Design review of the part built by this model. Coordinates are the model's own, in mm. Face numbers are marked on the shaded views. A direction names the side the tool comes from. Round coordinates to 2 decimals unless told otherwise and drop trailing zeros. Loops run counter-clockwise (first coordinate to the right, second up) from the corner with the lowest first, then second, coordinate; pieces in that order, holes last. Notation, with made-up numbers: (70.25, 68) -> (81.25, 68) arc R25 ccw to (81.25, 94) -> close; hole circle Ø1 at (20.5, 49.25). An arc over 180 degrees is marked (long way). Use a Markdown table: item, result. Add a question column.
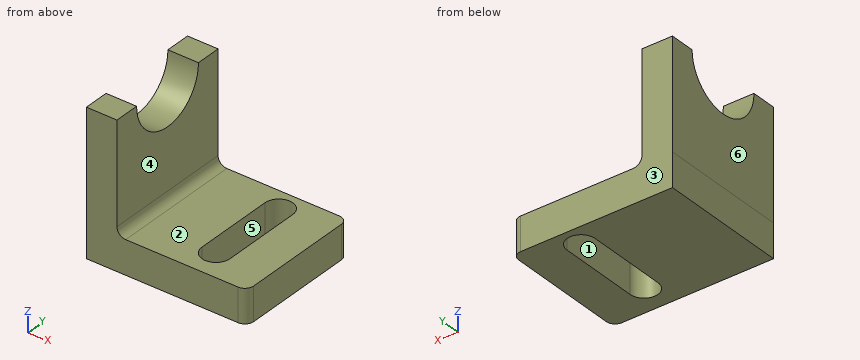
from build123d import *

# Parameters (mm, degrees)
F0_W     = 17.553337
F0_H     = 62.748581
F1_DEPTH = 75
F2_R     = 22.940745
F3_DEPTH = 25
F5_DEPTH = 19.308256
F6_R     = 5
F7_R     = 5


with BuildPart() as f1:
    # F0 (on Front) → F1 (new body)
    with BuildSketch(Plane.XZ):
        Polygon((-46.077821, -9.653628), (46.077821, -9.653628), (46.077821, 9.653628), (-28.524484, 9.653628), (-46.077821, 9.653628), align=None)
        with Locations((-37.301153, 41.027918)):
            Rectangle(F0_W, F0_H)
    extrude(amount=F1_DEPTH)

    # F2 (on face) → F3 (cut)
    with BuildSketch(Plane.YZ.offset(-28.524484)):
        with Locations((-37.5, 72.402209)):
            Circle(F2_R)
    extrude(amount=-F3_DEPTH, mode=Mode.SUBTRACT)

    # F4 (on face) → F5 (cut, through all)
    with BuildSketch(Plane.XY.offset(9.653628)):
        with BuildLine():
            Line((7.655139, -12.002843), (7.655139, -58.650463))
            ThreePointArc((7.655139, -58.650463), (15.655139, -66.650463), (23.655139, -58.650463))
            Line((23.655139, -58.650463), (23.655139, -12.002843))
            ThreePointArc((23.655139, -12.002843), (15.655139, -4.002843), (7.655139, -12.002843))
        make_face()
    extrude(amount=-F5_DEPTH, mode=Mode.SUBTRACT)

    # F6
    f6_edges = [f1.edges().sort_by_distance(p)[0] for p in [
        (46.077821, -75, 0),
        (46.077821, 0, 0),
    ]]
    fillet(f6_edges, radius=F6_R)

    # F7
    f7_edges = [f1.edges().sort_by_distance(p)[0] for p in [
        (-28.524484, -37.5, 9.653628),
    ]]
    fillet(f7_edges, radius=F7_R)


solid = f1.part
1. For the marked faces 1, 2 and 3, list the 3-axis set-ups (+Z, -Z, +X, -X, +Y, -Y) from which the entire face can be reached by the end or side of a thin tool; tool diameter is ignored.
2. Mouldability with a two-part tool opening along X and no side actions: class the marked faces 4, 5 and 6 as +X half, -X half, draft (parallel to the pull), parting line (faces both ways), or undercut.
3. Consider section B-B on x = -35. State the section outline as (y, z) points.
4. Insertion check: P1, Ø8, axis at x = -19, y = -15.5, coming from the +Z side; P2, Ø4, axis at x = -31, y = -25, coming from the +Z side; P3, Ø12, axis at y = -65.5, z = 19.5, coming from the +X side. Each pin has a flat end and moves straight along its axis. Give the tip position at first contact, or say it passes through.
5. Consider section C-C on y = -68. State the section outline as (x, z) points, plus the area to 3 significant figures.
6. Consider section A-A on y = -37.5. State the section outline as (x, z) points.
7. To check wall thickness, follow probe 1 along Z at (x, y) = (36.5, -72); probe 2 along X at (y, z) = (-57, 2.5); probe 3 along X at (y, z) = (-55.5, 26.5). State the ranges of each line that lie inside material, in increasing order. Write a range as from..to.
8. Consider section D-D on z = 42. State the section outline as (x, y) points.
Verdict:
| question | item | result |
|---|---|---|
| 1 | face 1 | +Z, -Z |
| 1 | face 2 | +Z, +X, +Y, -Y |
| 1 | face 3 | +Z, -Z, +X, -X, +Y |
| 2 | face 4 | +X half |
| 2 | face 5 | undercut |
| 2 | face 6 | -X half |
| 3 | outline | (-75, -9.65) -> (0, -9.65) -> (0, 72.4) -> (-14.56, 72.4) arc R22.94 cw to (-60.44, 72.4) -> (-75, 72.4) -> close |
| 4 | P1 | stops at z = 9.65 |
| 4 | P2 | stops at z = 54.63 |
| 4 | P3 | stops at x = -28.39 |
| 5 | outline | (-46.08, -9.65) -> (46.08, -9.65) -> (46.08, 9.65) -> (-23.52, 9.65) arc R5 cw to (-28.52, 14.65) -> (-28.52, 72.4) -> (-46.08, 72.4) -> close |
| 5 | area | 2,890 mm² |
| 6 | outline | (-46.08, -9.65) -> (7.66, -9.65) -> (7.66, 9.65) -> (-23.52, 9.65) arc R5 cw to (-28.52, 14.65) -> (-28.52, 49.46) -> (-46.08, 49.46) -> close; (23.66, -9.65) -> (46.08, -9.65) -> (46.08, 9.65) -> (23.66, 9.65) -> close |
| 7 | probe 1 | z = -9.65..9.65 |
| 7 | probe 2 | x = -46.08..7.66, 23.66..46.08 |
| 7 | probe 3 | x = -46.08..-28.52 |
| 8 | outline | (-46.08, -75) -> (-28.52, -75) -> (-28.52, 0) -> (-46.08, 0) -> close |
